The listing builds one solid part. Answer for the finished solid, in the listing's coordinates (mm). A direction names the side the tool comes from. Coordinates: 2 decimals unless noted, no trailing zeros. Order: outer loops, then holes, each group sorted by start corner. A loop starts at its lowest first (then second) coordinate and runs counter-clockwise, first axis right, second up.
```python
from build123d import *

# Parameters (mm, degrees)
F0_W      = 24
F0_H      = 19.22
F1_DEPTH  = 6
F3_DEPTH  = 6
F5_DEPTH  = 3.5
F6_W      = 24
F6_H      = 2.42
F7_DEPTH  = 0.25
F9_DEPTH  = 6
F11_DEPTH = 24
F12_R     = 0.15
F13_R     = 0.15


with BuildPart() as f1:
    # F0 (on Front) → F1 (new body)
    with BuildSketch(Plane.XZ):
        Rectangle(F0_W, F0_H)
    extrude(amount=-F1_DEPTH)

    # F2 (on face) → F3 (cut, through all)
    with BuildSketch(Plane.XZ):
        with BuildLine():
            ThreePointArc((-5.5, 6.11), (-5.93934, 7.17066), (-7, 7.61))
            Line((-7, 7.61), (-7, 6.11))
            Line((-7, 6.11), (-7, 4.61))
            ThreePointArc((-7, 4.61), (-5.93934, 5.04934), (-5.5, 6.11))
        make_face()
        with BuildLine():
            ThreePointArc((7, 7.61), (5.5, 6.11), (7, 4.61))
            Line((7, 4.61), (7, 6.11))
            Line((7, 6.11), (7, 7.61))
        make_face()
        with BuildLine():
            Line((7, 6.11), (7, 4.61))
            ThreePointArc((7, 4.61), (8.06066, 5.04934), (8.5, 6.11))
            ThreePointArc((8.5, 6.11), (8.06066, 7.17066), (7, 7.61))
            Line((7, 7.61), (7, 6.11))
        make_face()
        with BuildLine():
            ThreePointArc((7, 1.11), (5.93934, 0.67066), (5.5, -0.39))
            Line((5.5, -0.39), (7, -0.39))
            Line((7, -0.39), (7, 1.11))
        make_face()
        with BuildLine():
            Line((7, -0.39), (5.5, -0.39))
            ThreePointArc((5.5, -0.39), (7, -1.89), (8.5, -0.39))
            ThreePointArc((8.5, -0.39), (8.06066, 0.67066), (7, 1.11))
            Line((7, 1.11), (7, -0.39))
        make_face()
        with BuildLine():
            ThreePointArc((-5.5, -0.39), (-5.93934, 0.67066), (-7, 1.11))
            Line((-7, 1.11), (-7, -0.39))
            Line((-7, -0.39), (-5.5, -0.39))
        make_face()
        with BuildLine():
            Line((-7, -0.39), (-7, 1.11))
            ThreePointArc((-7, 1.11), (-8.06066, -1.45066), (-5.5, -0.39))
            Line((-5.5, -0.39), (-7, -0.39))
        make_face()
        with BuildLine():
            Line((-7, 6.11), (-7, 7.61))
            ThreePointArc((-7, 7.61), (-8.5, 6.11), (-7, 4.61))
            Line((-7, 4.61), (-7, 6.11))
        make_face()
    extrude(amount=-F3_DEPTH, mode=Mode.SUBTRACT)

    # F4 (on face) → F5 (cut)
    with BuildSketch(Plane.XZ):
        with BuildLine():
            ThreePointArc((-3.75, 6.11), (-7, 9.36), (-10.25, 6.11))
            Line((-10.25, 6.11), (-10.25, -0.39))
            ThreePointArc((-10.25, -0.39), (-7, -3.64), (-3.75, -0.39))
            Line((-3.75, -0.39), (-3.75, 6.11))
        make_face()
        with BuildLine():
            ThreePointArc((3.75, -0.39), (7, -3.64), (10.25, -0.39))
            Line((10.25, -0.39), (10.25, 6.11))
            ThreePointArc((10.25, 6.11), (7, 9.36), (3.75, 6.11))
            Line((3.75, 6.11), (3.75, -0.39))
        make_face()
    extrude(amount=-F5_DEPTH, mode=Mode.SUBTRACT)

    # F6 (on face) → F7 (cut)
    with BuildSketch(Plane.XZ):
        with Locations((0, -8.4)):
            Rectangle(F6_W, F6_H)
    extrude(amount=-F7_DEPTH, mode=Mode.SUBTRACT)

    # F8 (on face) → F9 (cut, through all)
    with BuildSketch(Plane.XZ):
        with BuildLine():
            ThreePointArc((-8.39, -4.89), (-8.495442, -4.635442), (-8.75, -4.53))
            Line((-8.75, -4.53), (-8.75, -4.89))
            Line((-8.75, -4.89), (-8.39, -4.89))
        make_face()
        with BuildLine():
            ThreePointArc((9.61, -4.89), (9.25, -4.53), (8.89, -4.89))
            ThreePointArc((8.89, -4.89), (9.25, -5.25), (9.61, -4.89))
        make_face()
        with BuildLine():
            ThreePointArc((5.61, -4.89), (5.25, -4.53), (4.89, -4.89))
            Line((4.89, -4.89), (5.25, -4.89))
            Line((5.25, -4.89), (5.61, -4.89))
        make_face()
        with BuildLine():
            Line((5.25, -4.89), (4.89, -4.89))
            ThreePointArc((4.89, -4.89), (5.25, -5.25), (5.61, -4.89))
            Line((5.61, -4.89), (5.25, -4.89))
        make_face()
        with BuildLine():
            ThreePointArc((-4.39, -4.89), (-4.75, -4.53), (-5.11, -4.89))
            Line((-5.11, -4.89), (-4.75, -4.89))
            Line((-4.75, -4.89), (-4.39, -4.89))
        make_face()
        with BuildLine():
            Line((-4.75, -4.89), (-5.11, -4.89))
            ThreePointArc((-5.11, -4.89), (-4.75, -5.25), (-4.39, -4.89))
            Line((-4.39, -4.89), (-4.75, -4.89))
        make_face()
        with BuildLine():
            Line((-8.75, -4.89), (-8.75, -4.53))
            ThreePointArc((-8.75, -4.53), (-9.004558, -5.144558), (-8.39, -4.89))
            Line((-8.39, -4.89), (-8.75, -4.89))
        make_face()
    extrude(amount=-F9_DEPTH, mode=Mode.SUBTRACT)

    # F10 (on face) → F11 (cut, through all)
    with BuildSketch(Plane.YZ.offset(12)):
        Polygon((2.2, -8.900258), (0.25, -9.61), (6, -9.61), (6, -8.900258), align=None)
    extrude(amount=-F11_DEPTH, mode=Mode.SUBTRACT)

    # F12
    f12_edges = [f1.edges().sort_by_distance(p)[0] for p in [
        (0, 0.25, -9.61),
    ]]
    fillet(f12_edges, radius=F12_R)

    # F13
    f13_edges = [f1.edges().sort_by_distance(p)[0] for p in [
        (0, 0.25, -7.19),
    ]]
    fillet(f13_edges, radius=F13_R)


solid = f1.part
```
1) A cutting plane is placed at C-C, the plane x = -6. Write down the section's boundary in (y, z).
2) A cutting plane is placed at A-A, the plane y = 3.95. Count the separate pieces of the cut face and the enclosed holes in it, plus the area to 3 significant figures.
3) For faces 1 (the flat face through (0, 6, 0)), 2 (the flat face through (0, 0.25, -8)), 3 (the flat face through (-10.25, 2, 3)), 4 (the flat face through (0, 4, -8.9)), determine the directions among +Z, -Z, +X, -X, +Y, -Y from which every point of the face is accessible in a straight line to the end or side of a thin tool.
4) Straight lines are drawn through the part: probe 1 along Z at (x, y) = (7, 4.2); probe 2 along X at (y, z) = (2.5, -4.89); probe 3 along X at (y, z) = (1.9, 0). For each, find the intervals that lie inside material, in ascending order.
5) Each of these flat-tipped pins is pushed along its axis until it touches: P1, Ø5, axis at x = -3.5, z = 3.5, coming from the -Y side; P2, Ø3, axis at x = -3.5, y = 3.5, coming from the -Z side; P3, Ø3, axis at x = -6.5, z = 4.5, coming from the -Y side. Where does it stop, or does it pass through?
6) A cutting plane is placed at B-B, the plane z = 3.5. Write down the section's boundary in (x, y).
7) A cutting plane is placed at D-D, the plane x = 9.25. Write down the section's boundary in (y, z).
8) The mould has two halves that part along X. Classify faces 5 (the flat face through (-12, 3, 0)), 6 (the flat face through (0, 3, 9.61)), 7 (the flat face through (-7, 3.5, 3)): released by +X, released by -X, zero draft, split by the parting line, or undercut.
Working result:
1. outline: (0, -7.19) - (0.1, -7.19) arc R0.15 cw to (0.25, -7.34) - (0.25, -9.4) arc R0.15 ccw to (0.45, -9.54) - (2.2, -8.9) - (6, -8.9) - (6, -1.51) - (3.5, -1.51) - (3.5, -3.48) - (0, -3.48) - close; (0, 9.2) - (3.5, 9.2) - (3.5, 7.23) - (6, 7.23) - (6, 9.61) - (0, 9.61) - close; (3.5, 0.73) - (6, 0.73) - (6, 4.99) - (3.5, 4.99) - close
2. separate pieces: 1
2. enclosed holes: 8
2. area: 414 mm2
3. face 1: +Z, -Z, +X, -X, +Y
3. face 2: -Z, +X, -X, -Y
3. face 3: -Y
3. face 4: -Z, +X, -X, +Y
4. probe 1: z = -8.9 to -1.89, 1.11 to 4.61, 7.61 to 9.61
4. probe 2: x = -12 to -9.11, -8.39 to -5.11, -4.39 to 4.89, 5.61 to 8.89, 9.61 to 12
4. probe 3: x = -12 to -10.25, -3.75 to 3.75, 10.25 to 12
5. P1: stops at y = 0
5. P2: stops at z = -8.97
5. P3: stops at y = 3.5
6. outline: (-12, 0) - (-10.25, 0) - (-10.25, 3.5) - (-3.75, 3.5) - (-3.75, 0) - (3.75, 0) - (3.75, 3.5) - (10.25, 3.5) - (10.25, 0) - (12, 0) - (12, 6) - (-12, 6) - close
7. outline: (0, -7.19) - (0.1, -7.19) arc R0.15 cw to (0.25, -7.34) - (0.25, -9.4) arc R0.15 ccw to (0.45, -9.54) - (2.2, -8.9) - (6, -8.9) - (6, -5.25) - (0, -5.25) - close; (0, -4.53) - (6, -4.53) - (6, 9.61) - (0, 9.61) - (0, 8.46) - (3.5, 8.46) - (3.5, -2.74) - (0, -2.74) - close
8. face 5: released by -X
8. face 6: zero draft
8. face 7: undercut
